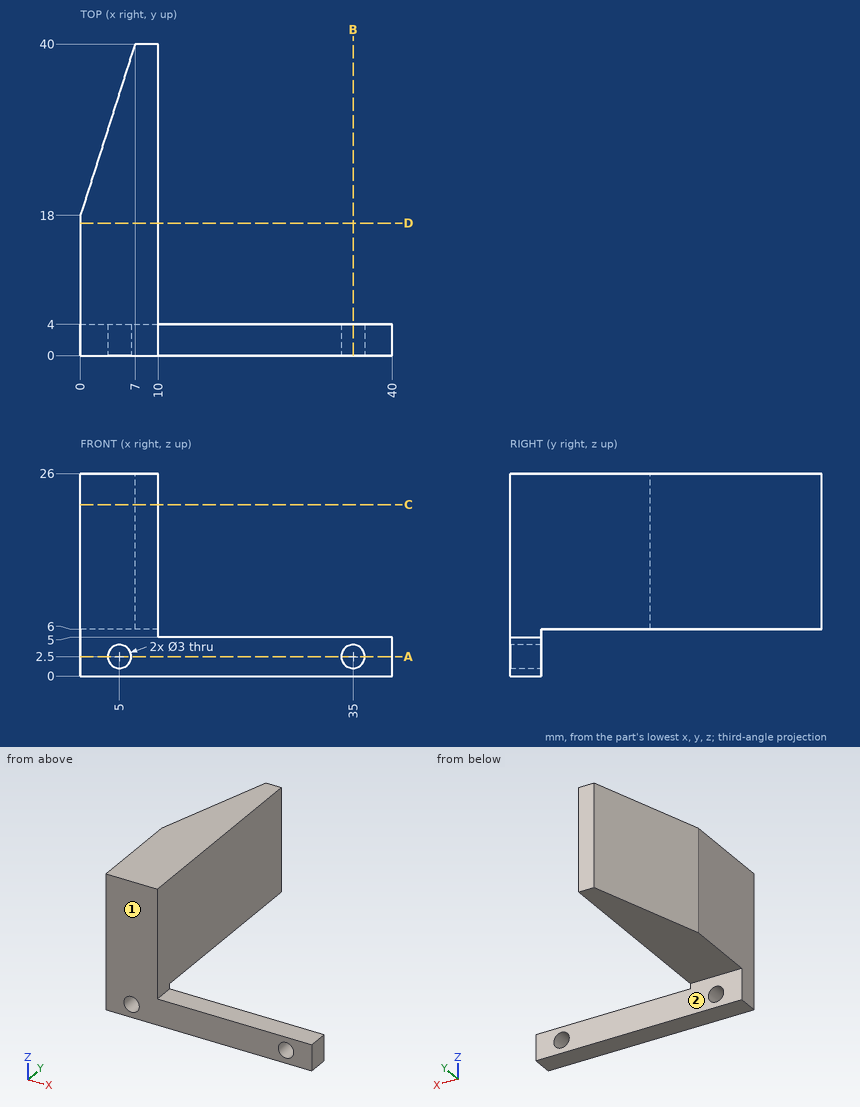
Job drawing, mm, ordinate dimensions from the low corner. One solid piece. A direction names the side the tool comes from. Round coordinates to 2 decimals unless told otherwise and drop trailing zeros. Write each loop counter-clockwise with the first axis right and the second up, starting at its lowest first coordinate (ties: lowest second). Pieces come first, ordered by that corner, then holes.
1) Band-saw the part on B-B, the plane x = 35. List the corners of the cut face in (y, z), and give its area (3 significant figures).
2) Band-saw the part on C-C, the plane z = 22. List the corners of the cut face in (x, y), and give its area (3 significant figures).
3) Band-saw the part on A-A, the plane z = 2.5. List the corners of the cut face in (x, y), and give its area (3 significant figures).
4) 3-axis set-ups, long thin cutter, end or side, ignore diameter. For the marked faces 1 and 2: which of +Z, -Z, +X, -X, +Y, -Y reach the whole face in a straight line?
5) Band-saw the part on D-D, the plane y = 17. List the corners of the cut face in (x, z), and give its area (3 significant figures).
6) Pin check, flat tips, straight feed: pin 1 (10 mm diameter, centred on y = 16, z = 11.5, fed in from +X); pin 2 (12 mm diameter, centred on x = 11, y = 13.5, fed in from -Z); pin 3 (1.8 mm diameter, centred on x = 11, z = 4, fed in from +Y). Stop position of each tip, or through.
7) Drill centre lines: probe 1 along X at (y, z) = (3.2, 2.5); probe 2 along Y at (x, z) = (24.5, 3.75); probe 3 along Z at (x, y) = (9, 12). Where is each one in solid material? Low to high.
Ans:
1. outline: (0, 0) - (4, 0) - (4, 1) - (0, 1) - close; (0, 4) - (4, 4) - (4, 5) - (0, 5) - close
1. area: 8.00 mm2
2. outline: (0, 0) - (10, 0) - (10, 40) - (7, 40) - (0, 18) - close
2. area: 323 mm2
3. outline: (0, 0) - (3.5, 0) - (3.5, 4) - (0, 4) - close; (6.5, 0) - (33.5, 0) - (33.5, 4) - (6.5, 4) - close; (36.5, 0) - (40, 0) - (40, 4) - (36.5, 4) - close
3. area: 136 mm2
4. face 1: +Z, -Z, +X, -X, -Y
4. face 2: -Z, +X, -X, +Y
5. outline: (0, 6) - (10, 6) - (10, 26) - (0, 26) - close
5. area: 200 mm2
6. pin 1: stops at x = 10
6. pin 2: stops at z = 6
6. pin 3: stops at y = 4
7. probe 1: x = 0 to 3.5, 6.5 to 33.5, 36.5 to 40
7. probe 2: y = 0 to 4
7. probe 3: z = 6 to 26
